from build123d import *

# Parameters (mm, degrees)
CROQUIS1_W              = 70
CROQUIS1_H              = 105
CROQUIS1_R              = 2
CROQUIS1_R_2            = 7.5
CROQUIS1_R_3            = 1.5
CROQUIS1_W_2            = 5.5
CROQUIS1_H_2            = 9
SALIENTE_EXTRUIR1_DEPTH = 5.5


with BuildPart() as part:
    # Croquis1 → Saliente-Extruir1 (new body)
    with BuildSketch(Plane(origin=(0, 0, 0), x_dir=(1, 0, 0), z_dir=(0, 1, 0))):
        with Locations((-71.406504065, -46.422764228)):
            Rectangle(CROQUIS1_W, CROQUIS1_H)
        with Locations(Location((-82.906504065, 1.077235772, 0), (0, 0, 270))):
            Circle(CROQUIS1_R, mode=Mode.SUBTRACT)
        with Locations(Location((-82.906504065, -27.922764228, 0), (0, 0, 270))):
            Circle(CROQUIS1_R, mode=Mode.SUBTRACT)
        with Locations(Location((-71.406504065, -43.922764228, 0), (0, 0, 270))):
            Circle(CROQUIS1_R_2, mode=Mode.SUBTRACT)
        with Locations(Location((-71.406504065, -8.922764228, 0), (0, 0, 270))):
            Circle(CROQUIS1_R_3, mode=Mode.SUBTRACT)
        with Locations(Location((-59.906504065, -27.922764228, 0), (0, 0, 90))):
            Circle(CROQUIS1_R, mode=Mode.SUBTRACT)
        with Locations(Location((-59.906504065, 1.077235772, 0), (0, 0, 90))):
            Circle(CROQUIS1_R, mode=Mode.SUBTRACT)
        with Locations(Location((-98.406504065, -8.922764228, 0), (0, 0, 270))):
            Circle(CROQUIS1_R_3, mode=Mode.SUBTRACT)
        with Locations(Location((-44.406504065, -8.922764228, 0), (0, 0, 90))):
            Circle(CROQUIS1_R_3, mode=Mode.SUBTRACT)
        with Locations((-83.656504065, -69.422764228)):
            Rectangle(CROQUIS1_W_2, CROQUIS1_H_2, mode=Mode.SUBTRACT)
        with Locations((-59.156504065, -69.422764228)):
            Rectangle(CROQUIS1_W_2, CROQUIS1_H_2, mode=Mode.SUBTRACT)
    extrude(amount=SALIENTE_EXTRUIR1_DEPTH)


solid = part.part
Read the model definition and answer for the solid it produces. Units are mm, in the model's axes. A direction names the side the tool comes from. Coordinates: 2 decimals unless noted, no trailing zeros. Write each loop counter-clockwise with the first axis right and the second up, starting at its lowest first coordinate (ties: lowest second). Pieces come first, ordered by that corner, then holes. Notation, with made-up numbers: (72.25, 33) -> (101.25, 33) arc R18 cw to (101.25, 62) -> close; hole circle Ø5 at (49, -11.5). An arc over 180 degrees is marked (long way). Return JSON: item names as keys, results as strings.
(1) The part is cut by section B-B on z = 50. Give the vertices of the cut face in (x, y).
Answers below:
{"outline": "(-106.41, 0) -> (-75.8, 0) -> (-75.8, 5.5) -> (-106.41, 5.5) -> close; (-67.01, 0) -> (-36.41, 0) -> (-36.41, 5.5) -> (-67.01, 5.5) -> close"}
(2) The part is cut by section A-A on z = 69.5. Give the vertices of the cut face in (x, y), then the cut area to 4 significant figures.
Answers below:
{"outline": "(-106.41, 0) -> (-86.41, 0) -> (-86.41, 5.5) -> (-106.41, 5.5) -> close; (-80.91, 0) -> (-61.91, 0) -> (-61.91, 5.5) -> (-80.91, 5.5) -> close; (-56.41, 0) -> (-36.41, 0) -> (-36.41, 5.5) -> (-56.41, 5.5) -> close", "area": "324.5 mm^2"}
(3) The part is cut by section C-C on y = 2.85. State how many separate pieces and enclosed holes the cut face has, then the cut area to 3 significant figures.
Answers below:
{"separate pieces": "1", "enclosed holes": "10", "area": "7,000 mm^2"}
(4) For a pull along Z with two mould halves and no side action, classify faces 3 (the flat face through (-80, 5.5, 46)), 4 (the flat face through (-72, 3, 98.923)), 5 (the cylindrical face through (-57.954, 2.712, -0.644)) as pulls with the +Z half, pulls with the -Z half, needs draft (parallel to the pull), parting line crosses it, or undercut.
Answers below:
{"face 3": "needs draft", "face 4": "pulls with the +Z half", "face 5": "undercut"}
(5) This flat-tipped pin is pushed along its axis until it touches: P1, Ø3.5, axis at x = -82.91, z = 27.92, coming from the -Y side. Where does it stop, or does it pass through?
Answers below:
{"P1": "through"}
(6) Which of the six approach directions +Z, -Z, +X, -X, +Y, -Y give full straight-line access (tool end or side, diameter ignored) to faces 1 (the flat face through (-59, 3, 64.923)), 2 (the flat face through (-106.407, 3, 47))?
Answers below:
{"face 1": "+Y, -Y", "face 2": "+Z, -Z, -X, +Y, -Y"}
(7) Consider line 1 along X through (y, z) = (2.35, 69); line 2 along X through (y, z) = (4.35, 28); line 3 along Z through (x, y) = (-61.5, 0.45). Determine where each line is inside the solid, lowest interval first. Write a range as from..to.
Answers below:
{"line 1": "-106.41..-86.41, -80.91..-61.91, -56.41..-36.41", "line 2": "-106.41..-84.91, -80.91..-61.91, -57.91..-36.41", "line 3": "-6.08..-2.29, 0.13..26.71, 29.13..64.92, 73.92..98.92"}
